CAD build for the part. Positions are in the model's coordinates, mm. A direction names the side the tool comes from. Give positions to 0.01 mm unless a question says otherwise; leave off trailing zeros. Order: outer loops, then holes, each group sorted by start corner. A loop starts at its lowest first (then second) coordinate and runs counter-clockwise, first axis right, second up. Notation, with made-up numbers: (71.5, 31.5) -> (127.5, 31.5) arc R27 cw to (127.5, 62.5) -> close; hole circle Ø4 at (35.25, 50.5). An arc over 180 degrees is marked (long way). Answer as CSV lines item,"result".
```python
from build123d import *

# Parameters (mm, degrees)
BOSS_EXTRU_1_DEPTH                              = 9
CHAMBRAGE_POUR_VIS_T_TE_CYLINDRIQUE_D           = 2.5
CHAMBRAGE_POUR_VIS_T_TE_CYLINDRIQUE_CBORE_D     = 4.5
CHAMBRAGE_POUR_VIS_T_TE_CYLINDRIQUE_CBORE_DEPTH = 1.5
CONG_1_R                                        = 0.5
ESQUISSE6_R                                     = 1.6
ENL_V_MAT_EXTRU_1_DEPTH                         = 19.27908646
ESQUISSE7_W                                     = 5.85
ESQUISSE7_H                                     = 2.25
ENL_V_MAT_EXTRU_2_DEPTH                         = 7.25


with BuildPart() as part:
    # Esquisse1 → Boss.-Extru.1 (new body)
    with BuildSketch(Plane(origin=(0, 0, 0), x_dir=(1, 0, 0), z_dir=(0, 1, 0))):
        with BuildLine():
            Line((6.025985397, 9.5), (-6.025985397, 9.5))
            ThreePointArc((-6.025985397, 9.5), (0, -11.25), (6.025985397, 9.5))
        make_face()
        with BuildLine():
            Line((-3.2, 0), (-3.2, 2.9))
            Line((-3.2, 2.9), (3.2, 2.9))
            Line((3.2, 2.9), (3.2, 0))
            ThreePointArc((3.2, 0), (0, -3.2), (-3.2, 0))
        make_face(mode=Mode.SUBTRACT)
    extrude(amount=BOSS_EXTRU_1_DEPTH)

    # Chambrage pour vis à tête cylindrique à 6 pans creux (ou vis CHC) M21 (through all)
    with Locations(Plane(origin=(0, 9, 0), x_dir=(1, 0, 0), z_dir=(0, 1, 0))):
        with Locations((8, 0), (-8, 0), (0, 0), (0, -8)):
            CounterBoreHole(CHAMBRAGE_POUR_VIS_T_TE_CYLINDRIQUE_D / 2, CHAMBRAGE_POUR_VIS_T_TE_CYLINDRIQUE_CBORE_D / 2, CHAMBRAGE_POUR_VIS_T_TE_CYLINDRIQUE_CBORE_DEPTH)

    # Congé1
    cong_1_edges = [part.edges().sort_by_distance(p)[0] for p in [
        (0, 9, 3.2),
        (3.2, 9, -1.45),
        (0, 9, -2.9),
        (-3.2, 9, -1.45),
    ]]
    fillet(cong_1_edges, radius=CONG_1_R)

    # Esquisse6 → Enlèv. mat.-Extru.1 (cut, through all)
    with BuildSketch(Plane.XY):
        with Locations((0, 5)):
            Circle(ESQUISSE6_R)
    extrude(amount=-ENL_V_MAT_EXTRU_1_DEPTH, mode=Mode.SUBTRACT)

    # Esquisse7 → Enlèv. mat.-Extru.2 (cut)
    with BuildSketch(Plane(origin=(0, 0, 0), x_dir=(1, 0, 0), z_dir=(0, 1, 0))):
        with Locations((0, 5.525)):
            Rectangle(ESQUISSE7_W, ESQUISSE7_H)
    extrude(amount=ENL_V_MAT_EXTRU_2_DEPTH, mode=Mode.SUBTRACT)


solid = part.part
```
1) Band-saw the part on B-B, the plane y = 1.75. Write the cut outline in (x, z) (3 decimals), then the cut area to 3 significant figures.
Data:
outline,"(-6.026, -9.5) -> (6.026, -9.5) arc R11.25 ccw (long way) to start; hole circle Ø2.5 at (-8, 0); hole (-3.2, -2.9) -> (3.2, -2.9) -> (3.2, 0) arc R3.2 ccw to (-3.2, 0) -> close; hole (-2.925, -6.65) -> (2.925, -6.65) -> (2.925, -4.4) -> (-2.925, -4.4) -> close; hole circle Ø2.5 at (0, 8); hole circle Ø2.5 at (8, 0)"
area,"321 mm2"
2) Pull direction Z, two halves, no side cores. Call faces 5 (the cylindrical face through (-0.406, 4.437, 11.243)), 6 (the flat face through (2, 0, 3)), 7 (the flat face through (-7, 7.5, 1)): pulls with the +Z half, pulls with the -Z half, needs draft (parallel to the pull), parting line crosses it, or undercut.
Data:
face 5,"parting line crosses it"
face 6,"needs draft"
face 7,"undercut"
3) Band-saw the part on C-C, the plane z = 8. Write the cut outline in (x, y).
Data:
outline,"(-7.91, 0) -> (-1.25, 0) -> (-1.25, 7.5) -> (-2.25, 7.5) -> (-2.25, 9) -> (-7.91, 9) -> close; (1.25, 0) -> (7.91, 0) -> (7.91, 9) -> (2.25, 9) -> (2.25, 7.5) -> (1.25, 7.5) -> close"
4) Band-saw the part on D-D, the plane y = 5. Write the cut outline in (x, z) (3 decimals), then the cut area to 3 significant figures.
Data:
outline,"(-6.026, -9.5) -> (-1.6, -9.5) -> (-1.6, -6.65) -> (-2.925, -6.65) -> (-2.925, -4.4) -> (-1.6, -4.4) -> (-1.6, -2.9) -> (-3.2, -2.9) -> (-3.2, 0) arc R3.2 cw to (3.2, 0) -> (3.2, -2.9) -> (1.6, -2.9) -> (1.6, -4.4) -> (2.925, -4.4) -> (2.925, -6.65) -> (1.6, -6.65) -> (1.6, -9.5) -> (6.026, -9.5) arc R11.25 ccw (long way) to start; hole circle Ø2.5 at (-8, 0); hole circle Ø2.5 at (0, 8); hole circle Ø2.5 at (8, 0)"
area,"307 mm2"
5) Band-saw the part on A-A, the plane x = 0. Give the number of separate pieces and of enclosed holes in the cut face, then the cut area to 3 significant figures.
Data:
separate pieces,"5"
enclosed holes,"0"
area,"76.0 mm2"
6) Pin check, flat tips, straight feed: P1, Ø3.5, axis at x = 8, z = 0, coming from the +Y side; P2, Ø1, axis at y = 7.5, z = -6, coming from the +X side; P3, Ø5, axis at x = 3.5, y = 4, coming from the +Z side. Stop position of each tip, or through.
Data:
P1,"stops at y = 7.5"
P2,"stops at x = 9.81"
P3,"stops at z = 11.21"
7) Wall check: line 1 along Z through (x, y) = (-2.25, 3.5); line 2 along X through (y, z) = (8.25, 1.5); line 3 along Z through (x, y) = (-2.75, 4.25). Give the ranges that are in metal, low to high. Write a range as [from, to].
Data:
line 1,"z = [-9.5, -6.65], [-4.4, -2.9], [2.28, 11.02]"
line 2,"x = [-11.15, -9.68], [-6.32, -2.83], [2.83, 6.32], [9.68, 11.15]"
line 3,"z = [-9.5, -6.65], [-4.4, -2.9], [1.64, 10.91]"
8) Which spindle directions (+Z, -Z, +X, -X, +Y, -Y) get a long thin tool onto all of the face, cutting with end or side? Do faces 1 (the flat face through (3.2, 4, -1)), 2 (the cylindrical face through (-0.35, 3.44, -8.06)), 3 (the flat face through (0, 3, -6.65)), 4 (the cylindrical face through (-10.248, 8.26, -0.099)). Say none if no direction does.
Data:
face 1,"+Y, -Y"
face 2,"-Z"
face 3,"-Y"
face 4,"+Y"
